Input: part model. Units: mm. Frame: model coordinates. A direction names the side the tool comes from. Give positions to 0.01 mm unless a question says otherwise; leave off trailing zeros. Loops run counter-clockwise (first coordinate to the right, second up) from the corner with the lowest first, then second, coordinate; pieces in that order, holes last. Notation, with made-up numbers: (74, 88.25) - (94, 88.25) arc R12 ccw to (94, 106.25) - close; hole circle Ø9 at (-30.5, 42). An arc over 180 degrees is marked (long way). Answer as a JSON object with one key per item and string values. Group by question number.
(1) Section query B-B (x = 0). Return loops of the section in (y, z) (3 decimals).
(2) Access query for faces 1 (the flat face through (-15, 0, 1)), 2 (the cylindrical face through (-14.507, -11.446, 18.604)), 3 (the cylindrical face through (14.507, -12.765, 15.528)). Directions: +Z, -Z, +X, -X, +Y, -Y. A direction counts if a zero-diameter tool reaches every point of the face in a straight line with its end or side. Return the directions, or none.
(3) Section query C-C (y = 7.25). Return loops of the section in (x, z), plus the area to 3 significant figures.
(4) Section query A-A (z = -25). Return loops of the section in (x, y) (3 decimals), plus the area to 3 significant figures.
(5) Material intervals for L1, parallel to Z at x = 0, y = -4.75; L2, parallel to Z at x = -14.3, y = 0; L3, parallel to X at y = 4, z = 55, sorted ascending.
(6) Section query D-D (z = 15). Return loops of the section in (x, y), plus the area to 3 significant figures.
(7) Mould query, pull axis Y, two halves, no side actions, for faces 4 (the cylindrical face through (-0.2, 13.5, -10)), 5 (the flat face through (-14, 0, 15)), 6 (the flat face through (0, -14, 1)), 7 (the flat face through (0, 0, -65)). Classes: +Y half, -Y half, draft (parallel to the pull), parting line (faces both ways), or undercut.
```python
from build123d import *

# Parameters (mm, degrees)
SKETCH_1_W                        = 30
SKETCH_1_H                        = 28
EXTRUDE_1_DEPTH                   = 65
SKETCH_2_R                        = 2.5
CUT_EXTRUDE_1_DEPTH               = 73.945184899
HOLE_WIZARD_8_0_8_1_D             = 8
HOLE_WIZARD_8_0_8_1_CSINK_D       = 8.05
HOLE_WIZARD_8_0_8_1_CSINK_ANGLE   = 90
HOLE_WIZARD_10_0_10_1_D           = 10
HOLE_WIZARD_10_0_10_1_CSINK_D     = 10.05
HOLE_WIZARD_10_0_10_1_CSINK_ANGLE = 90
SKETCH_7_R                        = 12
CUT_EXTRUDE_2_DEPTH               = 1
SKETCH_9_R                        = 12
CUT_EXTRUDE_3_DEPTH               = 1


with BuildPart() as part:
    # 草图1 → 凸台-拉伸1 (new, symmetric)
    with BuildSketch(Plane.XY):
        Rectangle(SKETCH_1_W, SKETCH_1_H)
    extrude(amount=EXTRUDE_1_DEPTH, both=True)

    # 草图2 → 切除-拉伸1 (cut, through all)
    with BuildSketch(Plane.ZY.offset(15)):
        with Locations((-10, 16)):
            Circle(SKETCH_2_R)
    extrude(amount=-CUT_EXTRUDE_1_DEPTH, mode=Mode.SUBTRACT)

    # Ø8.0 (8) 直径孔1 (through all)
    with Locations(Plane(origin=(0, 14, 0), x_dir=(1, 0, 0), z_dir=(0, 1, 0))):
        with Locations((0, 25), (0, 50)):
            CounterSinkHole(HOLE_WIZARD_8_0_8_1_D / 2, HOLE_WIZARD_8_0_8_1_CSINK_D / 2, counter_sink_angle=HOLE_WIZARD_8_0_8_1_CSINK_ANGLE)

    # Ø10.0 (10) 直径孔1 (through all)
    with Locations(Plane(origin=(0, 14, 0), x_dir=(1, 0, 0), z_dir=(0, 1, 0))):
        with Locations((0, -55)):
            CounterSinkHole(HOLE_WIZARD_10_0_10_1_D / 2, HOLE_WIZARD_10_0_10_1_CSINK_D / 2, counter_sink_angle=HOLE_WIZARD_10_0_10_1_CSINK_ANGLE)

    # 草图7 → 切除-拉伸2 (cut)
    with BuildSketch(Plane.ZY.offset(15)):
        with Locations(Location((15, 0, 0), (0, 0, 270))):
            Circle(SKETCH_7_R)
    extrude(amount=-CUT_EXTRUDE_2_DEPTH, mode=Mode.SUBTRACT)

    # 草图9 → 切除-拉伸3 (cut)
    with BuildSketch(Plane(origin=(15, 0, 0), x_dir=(0, 0, -1), z_dir=(1, 0, 0))):
        with Locations(Location((-15, -0.777034021, 0), (0, 0, 90))):
            Circle(SKETCH_9_R)
    extrude(amount=-CUT_EXTRUDE_3_DEPTH, mode=Mode.SUBTRACT)


solid = part.part
```
Recorded:
{
 "1": {"outline": "(-14, -65) - (14, -65) - (14, -54.025) - (13.975, -54) - (-14, -54) - close; (-14, -46) - (13.975, -46) - (14, -45.975) - (14, -29.025) - (13.975, -29) - (-14, -29) - close; (-14, -21) - (13.975, -21) - (14, -20.975) - (14, -11.5) arc R2.5 cw to (14, -8.5) - (14, 49.975) - (13.975, 50) - (-14, 50) - close; (-14, 60) - (13.975, 60) - (14, 60.025) - (14, 65) - (-14, 65) - close"},
 "2": {"face 1": "+Z, -Z, -X, +Y, -Y", "face 2": "-X", "face 3": "+X"},
 "3": {"outline": "(-15, -65) - (15, -65) - (15, 6.08) - (14, 6.08) - (14, 23.92) - (15, 23.92) - (15, 65) - (-15, 65) - (-15, 24.56) - (-14, 24.56) - (-14, 5.44) - (-15, 5.44) - close; hole circle Ø10 at (0, 55); hole circle Ø8 at (0, -50); hole circle Ø8 at (0, -25)", "area": "3,680 mm^2"},
 "4": {"outline": "(-15, -14) - (-4, -14) - (-4, 13.975) - (-4.025, 14) - (-15, 14) - close; (4, -14) - (15, -14) - (15, 14) - (4.025, 14) - (4, 13.975) - close", "area": "616 mm^2"},
 "5": {"L1": "z = -65 to -54, -46 to -29, -21 to 50, 60 to 65", "L2": "z = -65 to 3, 27 to 65", "L3": "x = -15 to -5, 5 to 15"},
 "6": {"outline": "(-15, -14) - (15, -14) - (15, -12.78) - (14, -12.78) - (14, 11.22) - (15, 11.22) - (15, 14) - (-15, 14) - (-15, 12) - (-14, 12) - (-14, -12) - (-15, -12) - close", "area": "792 mm^2"},
 "7": {"face 4": "+Y half", "face 5": "undercut", "face 6": "-Y half", "face 7": "draft"}
}
